from build123d import *

# Parameters (mm, degrees)
BOSS_EXTRUDE1_DEPTH = 155
BOSS_EXTRUDE2_DEPTH = 66
BOSS_EXTRUDE3_DEPTH = 313
BOSS_EXTRUDE4_DEPTH = 54
BOSS_EXTRUDE5_DEPTH = 88
BOSS_EXTRUDE6_DEPTH = 41
BOSS_EXTRUDE7_DEPTH = 164
BOSS_EXTRUDE8_DEPTH = 63


with BuildPart() as part:
    # Sketch1 → Boss-Extrude1 (new body)
    with BuildSketch(Plane.XY):
        Polygon((-220.063797357, 0), (-198.907917785, -153.12825629), (-173.722346865, -226.670123376), (-10.519847306, -189.899189833), (-10.519847306, -270.996728194), (6.417174186, -320.452830951), (77.125939495, -337.486635422), (132.857093021, -303.394090716), (145.53009844, -250.787371679), (94.572304418, -167.486560125), (164.014799865, -143.704883603), (180.076897751, -110.911433751), (196.900067844, -76.564128145), (196.900067844, 0), align=None)
    boss_extrude1 = extrude(amount=BOSS_EXTRUDE1_DEPTH)

    # Sketch2 → Boss-Extrude2 (add)
    with BuildSketch(Plane.XY.offset(155)):
        Polygon((-220.063797357, 0), (-198.907917785, -153.12825629), (-173.722346865, -226.670123376), (164.014799865, -143.704883603), (196.900067844, -76.564128145), (196.900067844, 0), align=None)
    boss_extrude2 = extrude(amount=BOSS_EXTRUDE2_DEPTH)

    # Sketch3 → Boss-Extrude3 (add)
    with BuildSketch(Plane.XY.offset(221)):
        Polygon((-220.063797357, 0), (-198.907917785, -153.12825629), (-173.722346865, -226.670123376), (-144.188560723, -219.415139219), (-72.64388975, -185.187503489), (-13.784604036, -148.831636487), (0, -104.745103877), (6.910898911, -82.642360162), (38.419722404, -82.642360162), (117.796003981, -44.66800911), (131.76241917, 0), align=None)
    boss_extrude3 = extrude(amount=BOSS_EXTRUDE3_DEPTH)

    # Sketch4 → Boss-Extrude4 (add)
    with BuildSketch(Plane.XY.offset(534)):
        Polygon((-220.063797357, 0), (-163.514117876, -191.576655197), (-139.411479093, -184.462027915), (-116.05966541, -85.56138905), (-66.585874541, -85.56138905), (-31.247452492, -59.309989814), (78.107863193, -63.655184636), (117.796003981, -44.66800911), (131.76241917, 0), align=None)
    boss_extrude4 = extrude(amount=BOSS_EXTRUDE4_DEPTH)

    # Sketch5 → Boss-Extrude5 (add)
    with BuildSketch(Plane.XY.offset(588)):
        Polygon((-189.830764245, 0), (-173.676057022, -71.426020231), (-72.709136882, -71.426020231), (-44.150689094, -42.867572442), (-44.150689094, 0), align=None)
    boss_extrude5 = extrude(amount=BOSS_EXTRUDE5_DEPTH)

    # Sketch6 → Boss-Extrude6 (add)
    with BuildSketch(Plane.XY.offset(676)):
        with BuildLine():
            Line((-135.243392737, 0), (-124.137031521, -30.029582973))
            Line((-124.137031521, -30.029582973), (-67.595556243, -38.106936584))
            Line((-67.595556243, -38.106936584), (-9.982142183, -34.068259779))
            ThreePointArc((-9.982142183, -34.068259779), (-10.876517561, -17.044564178), (-11.174764407, 0))
            Line((-11.174764407, 0), (-135.243392737, 0))
        make_face()
    boss_extrude6 = extrude(amount=BOSS_EXTRUDE6_DEPTH)

    # Sketch7 → Boss-Extrude7 (add)
    with BuildSketch(Plane.XY.offset(717)):
        with BuildLine():
            Line((-102.933978292, 0), (-94.85662468, -28.01024457))
            Line((-94.85662468, -28.01024457), (-44.150689094, -39.665516705))
            Line((-44.150689094, -39.665516705), (-7.961701602, -39.665516705))
            ThreePointArc((-7.961701602, -39.665516705), (83.027852783, -78.239664369), (143.40681265, 0))
            Line((143.40681265, 0), (-7.961701602, 0))
            Line((-7.961701602, 0), (-102.933978292, 0))
        make_face()
    boss_extrude7 = extrude(amount=BOSS_EXTRUDE7_DEPTH)

    # Sketch8 → Boss-Extrude8 (add)
    with BuildSketch(Plane(origin=(0, 0, 0), x_dir=(-1, 0, 0), z_dir=(0, 0, -1))):
        with BuildLine():
            Line((-156.103280221, 0), (156.103280221, 0))
            ThreePointArc((156.103280221, 0), (0, -156.103280221), (-156.103280221, 0))
        make_face()
    boss_extrude8 = extrude(amount=BOSS_EXTRUDE8_DEPTH)

    # Mirror1: Boss-Extrude1, Boss-Extrude2, Boss-Extrude3, Boss-Extrude4, Boss-Extrude5, Boss-Extrude6, Boss-Extrude7, Boss-Extrude8 across plane
    add(boss_extrude1.mirror(Plane(origin=(196.900067844, 0, 155), x_dir=(0, 0, 1), z_dir=(0, -1, 0))))
    add(boss_extrude2.mirror(Plane(origin=(196.900067844, 0, 155), x_dir=(0, 0, 1), z_dir=(0, -1, 0))))
    add(boss_extrude3.mirror(Plane(origin=(196.900067844, 0, 155), x_dir=(0, 0, 1), z_dir=(0, -1, 0))))
    add(boss_extrude4.mirror(Plane(origin=(196.900067844, 0, 155), x_dir=(0, 0, 1), z_dir=(0, -1, 0))))
    add(boss_extrude5.mirror(Plane(origin=(196.900067844, 0, 155), x_dir=(0, 0, 1), z_dir=(0, -1, 0))))
    add(boss_extrude6.mirror(Plane(origin=(196.900067844, 0, 155), x_dir=(0, 0, 1), z_dir=(0, -1, 0))))
    add(boss_extrude7.mirror(Plane(origin=(196.900067844, 0, 155), x_dir=(0, 0, 1), z_dir=(0, -1, 0))))
    add(boss_extrude8.mirror(Plane(origin=(196.900067844, 0, 155), x_dir=(0, 0, 1), z_dir=(0, -1, 0))))


solid = part.part
Check sheet for the modelled part. Datum: model origin and axes. Units: mm. A direction names the side the tool comes from. Round coordinates to 2 decimals unless told otherwise and drop trailing zeros. Order: outer loops, then holes, each group sorted by start corner. A loop starts at its lowest first (then second) coordinate and runs counter-clockwise, first axis right, second up.
Q1. Scan lines: L1, parallel to Z at x = 25.5, y = 28.5; L2, parallel to Z at x = 149, y = -53; L3, parallel to Z at x = -150, y = 127. Record each from-to range of solid material in increasing order.
Filled sheet:
L1: z = -63 to 588, 717 to 881
L2: z = 0 to 221
L3: z = 0 to 588
Q2. Draft check along Z on faces 4 (the face through (-27, -1, 676)), 5 (the face through (46, -1, 881)), 6 (the face through (-26, -39.666, 798)). Enter one of: pulls with the +Z half, pulls with the -Z half, needs draft (parallel to the pull), parting line crosses it, or undercut.
Filled sheet:
face 4: undercut
face 5: pulls with the +Z half
face 6: needs draft
Q3. Cross-section at A-A, the plane x = 17.5. Enter the section's corners in (y, z), plus the area to 3 significant figures.
Filled sheet:
outline: (-323.12, 0) - (-155.12, 0) - (-155.12, -63) - (155.12, -63) - (155.12, 0) - (323.12, 0) - (323.12, 155) - (179.7, 155) - (179.7, 221) - (82.64, 221) - (82.64, 534) - (61.25, 534) - (61.25, 588) - (-61.25, 588) - (-61.25, 534) - (-82.64, 534) - (-82.64, 221) - (-179.7, 221) - (-179.7, 155) - (-323.12, 155) - close; (-67.19, 717) - (67.19, 717) - (67.19, 881) - (-67.19, 881) - close
area: 224,000 mm2
Q4. Set-up check for faces 1 (the face through (124.68, 22.65, 401.93)), 2 (the face through (-192.2, -94.4, 560.6)), 3 (the face through (128.81, 155.76, 76.41)): record each of +Z, -Z, +X, -X, +Y, -Y from which the full face is reachable in a straight line by a thin tool's end or side.
Filled sheet:
face 1: +X, +Y
face 2: +Z, -X, -Y
face 3: +Z, -Z, +X
Q5. Depth check by flat-ended pin: P1, Ø5, axis at x = 137.5, y = -265.5, coming from the -Z side; P2, Ø4, axis at x = -87, z = 54.5, coming from the -Y side; P3, Ø2, axis at x = 45.5, z = 51.5, coming from the +Y side. Enter the tip coordinate at first touch or a pass-through.
Filled sheet:
P1: stops at z = 0
P2: stops at y = -207.58
P3: stops at y = 330.11
